The drawing under review shows one solid part. Ordinate dimensions are in mm from its lowest x, y, z. Round coordinates to 2 decimals unless told otherwise and drop trailing zeros. Order: outer loops, then holes, each group sorted by start corner. A loop starts at its lowest first (then second) coordinate and runs counter-clockwise, first axis right, second up.
1) Consider section B-B (z = 13.5). Give the boundary of the cut face in (x, y).
2) Consider section C-C (z = 23.25). Give the boundary of the cut face in (x, y).
3) To check wall thickness, follow L1, parallel to Y at x = 15, z = 2.75; L2, parallel to Z at x = 14, y = 26; L3, parallel to X at y = 29, z = 1.5. State the ranges of each line that lie inside material, in increasing order.
4) Consider section D-D (y = 34.5). Give the boundary of the cut face in (x, z).
5) Consider section A-A (x = 15.25). Give the boundary of the cut face in (y, z).
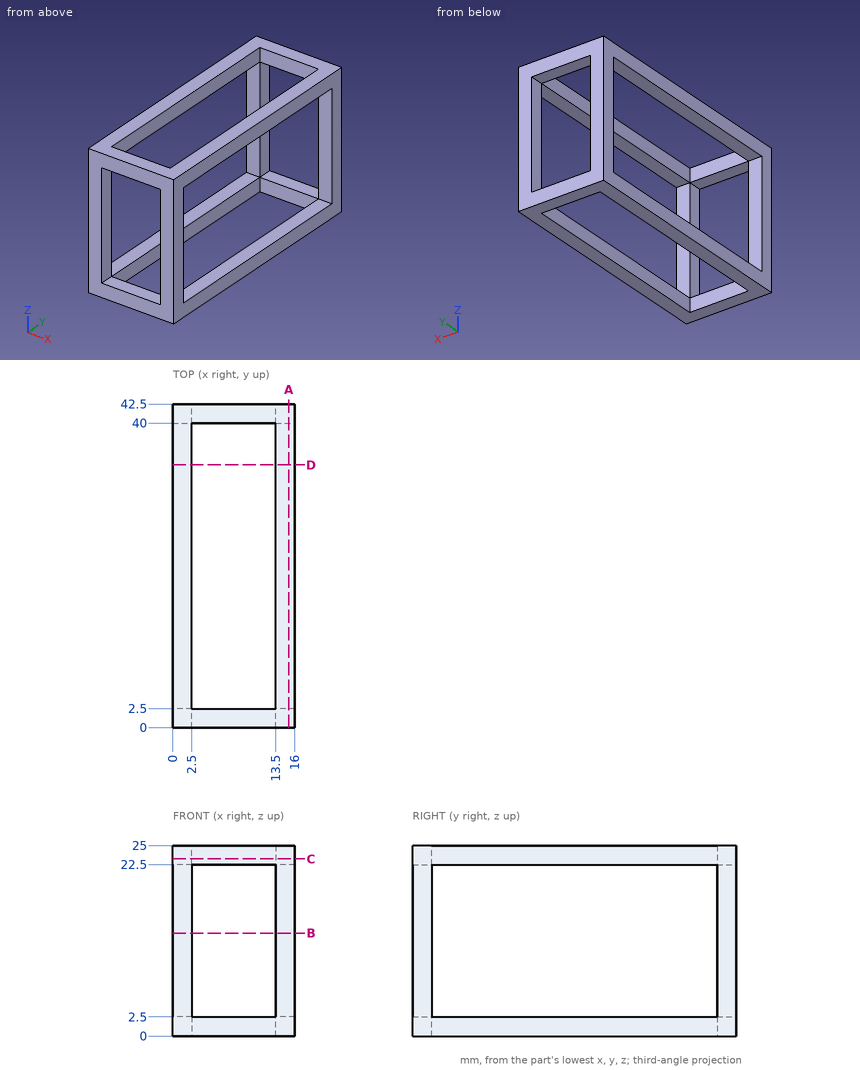
Answer below:
1. outline: (0, 0) - (2.5, 0) - (2.5, 2.5) - (0, 2.5) - close; (0, 40) - (2.5, 40) - (2.5, 42.5) - (0, 42.5) - close; (13.5, 0) - (16, 0) - (16, 2.5) - (13.5, 2.5) - close; (13.5, 40) - (16, 40) - (16, 42.5) - (13.5, 42.5) - close
2. outline: (0, 0) - (16, 0) - (16, 42.5) - (0, 42.5) - close; hole (2.5, 2.5) - (13.5, 2.5) - (13.5, 40) - (2.5, 40) - close
3. L1: y = 0 to 2.5, 40 to 42.5
3. L2: z = 0 to 2.5, 22.5 to 25
3. L3: x = 0 to 2.5, 13.5 to 16
4. outline: (0, 0) - (2.5, 0) - (2.5, 2.5) - (0, 2.5) - close; (0, 22.5) - (2.5, 22.5) - (2.5, 25) - (0, 25) - close; (13.5, 0) - (16, 0) - (16, 2.5) - (13.5, 2.5) - close; (13.5, 22.5) - (16, 22.5) - (16, 25) - (13.5, 25) - close
5. outline: (0, 0) - (42.5, 0) - (42.5, 25) - (0, 25) - close; hole (2.5, 2.5) - (40, 2.5) - (40, 22.5) - (2.5, 22.5) - close
